Can you work these out from the drawing? Everything is in mm from the part's minimum corner. A direction names the side the tool comes from. Coordinates: 2 decimals unless noted, no trailing zeros. Loops run counter-clockwise (first coordinate to the right, second up) from the corner with the lowest first, then second, coordinate; pieces in that order, holes last. Notation, with made-up numbers: (-16, -17) -> (3, -17) arc R22 cw to (3, -6) -> close; hole circle Ø6 at (7, 46). An arc over 180 degrees is marked (long way). Use one line per item in the form item = value. Start each with the question number.
(1) Imagine slicing it at D-D (y = 16). List the corners of the cut face in (x, z) for me.
(2) On a 3-axis mill with a long thin cutter (end or side, diameter ignored), from which of +Z, -Z, +X, -X, +Y, -Y can I reach the whole of each face in a straight line? I mean the marked faces 1, 2, 3 and 4. Say none if no direction works.
(3) Thinking about a two-plate mould opening in Y: for the marked faces 5, 6 and 7, which applies, released by +Y, released by -Y, zero draft, split by the parting line, or undercut?
(4) I need wall thicknesses on line 1 (Y direction, x = 39.5, z = 16.5); line 2 (X direction, y = 74, z = 73); line 3 (Y direction, x = 63, z = 146.5). Which ranges of each line are inside material? Lowest first, please. Write a range as [from, to].
(5) Imagine slicing it at A-A (x = 47). List the corners of the cut face in (y, z) for me, plus the area to 3 significant figures.
(6) Imagine slicing it at B-B (z = 65.5). List the corners of the cut face in (x, y) for me.
(7) I'm going to push flat-ended pins straight in: pin 1 (5 mm diameter, centred on y = 25, z = 64.5, fed in from -X); pin 2 (5.5 mm diameter, centred on x = 95.5, y = 57.5, fed in from +Z); pin 3 (1 mm diameter, centred on y = 86.5, z = 103.5, fed in from +X). Where does each tip first touch, or does it pass through?
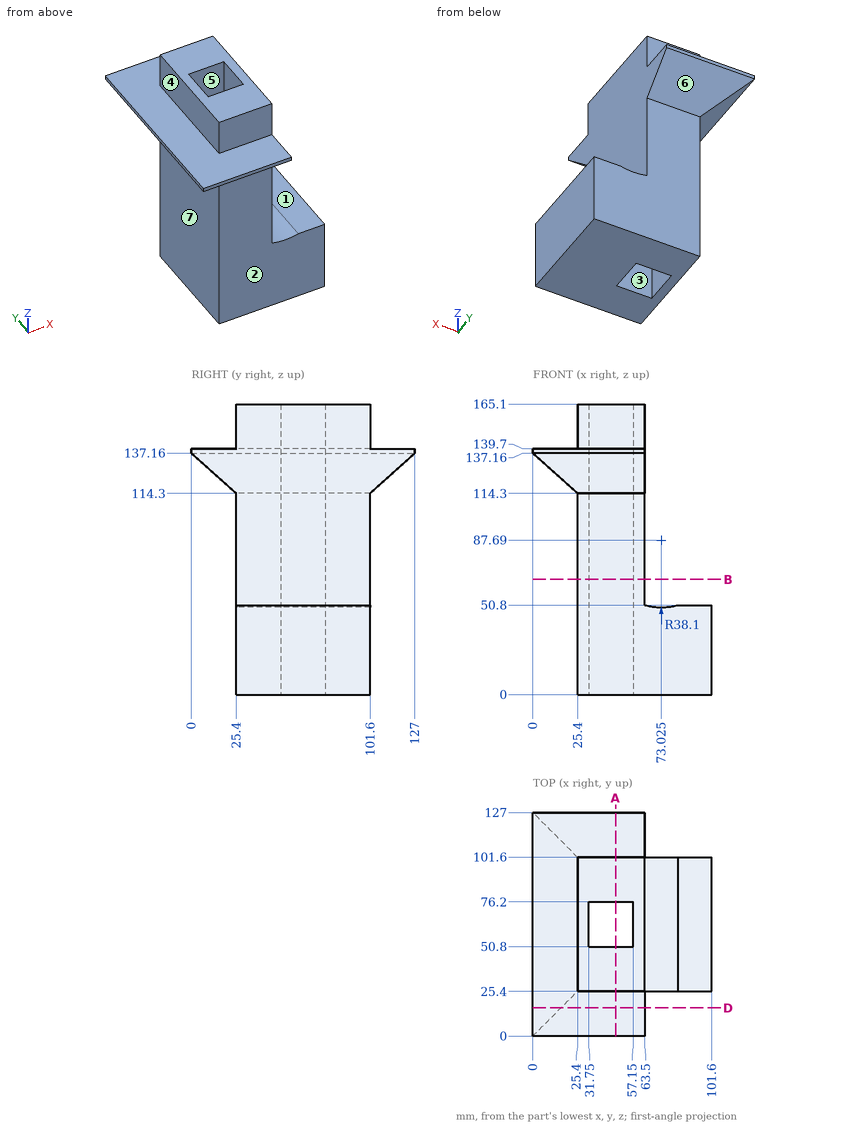
Worked out:
q1.outline = (0, 137.16) -> (16, 122.76) -> (63.5, 122.76) -> (63.5, 139.7) -> (0, 139.7) -> close
q2.face_1 = +Z, +X, +Y, -Y
q2.face_2 = -Z, +X, -X, -Y
q2.face_3 = +Z, -Z
q2.face_4 = +Z, -X, +Y, -Y
q3.face_5 = undercut
q3.face_6 = released by +Y
q3.face_7 = zero draft
q4.line_1 = [25.4, 50.8], [76.2, 101.6]
q4.line_2 = [25.4, 31.75], [57.15, 63.5]
q4.line_3 = [25.4, 101.6]
q5.outline = (0, 137.16) -> (25.4, 114.3) -> (25.4, 0) -> (50.8, 0) -> (50.8, 165.1) -> (25.4, 165.1) -> (25.4, 139.7) -> (0, 139.7) -> close; (76.2, 0) -> (101.6, 0) -> (101.6, 114.3) -> (127, 137.16) -> (127, 139.7) -> (101.6, 139.7) -> (101.6, 165.1) -> (76.2, 165.1) -> close
q5.area = 9,100 mm2
q6.outline = (25.4, 25.4) -> (63.5, 25.4) -> (63.5, 101.6) -> (25.4, 101.6) -> close; hole (31.75, 50.8) -> (57.15, 50.8) -> (57.15, 76.2) -> (31.75, 76.2) -> close
q7.pin_1 = 25.4
q7.pin_2 = 50.8
q7.pin_3 = 63.5
